from build123d import *

# Parameters (mm, degrees)
F0_W      = 120
F0_H      = 15
F1_DEPTH  = 781
F3_W      = 8
F3_H      = 8
F5_W      = 55
F5_H      = 12
F6_DEPTH  = 25
F7_W      = 20
F7_H      = 32
F9_DEPTH  = 25
F8_W      = 20
F8_H      = 32
F10_DEPTH = 25
F11_R     = 5


with BuildPart() as f1:
    # F0 (on Right) → F1 (new body)
    with BuildSketch(Plane.YZ):
        Rectangle(F0_W, F0_H)
    extrude(amount=F1_DEPTH)

    # F4: sweep along a path in F2
    with BuildLine(Plane.XY.offset(7.5)) as f4_path:
        Line((153, 60), (153, 10))
        ThreePointArc((153, 10), (155.928932, 2.928932), (163, 0))
        Line((163, 0), (553, 0))
        ThreePointArc((553, 0), (560.071068, 2.928932), (563, 10))
        Line((563, 10), (563, 60))
    # F3 (on face) → F4 (sweep, cut)
    with BuildSketch(Plane(origin=(0, 60, 0), x_dir=(-1, 0, 0), z_dir=(0, 1, 0))):
        with Locations((-152.987316, 11.5)):
            Rectangle(F3_W, F3_H)
        with Locations((-152.987316, 3.5)):
            Rectangle(F3_W, F3_H)
    sweep(path=f4_path.line, mode=Mode.SUBTRACT)

    # F5 (on face) → F6 (cut)
    with BuildSketch(Plane.XY.offset(7.5)):
        with Locations((152.987316, 60)):
            Rectangle(F5_W, F5_H)
        with Locations((563.012684, 60)):
            Rectangle(F5_W, F5_H)
    extrude(amount=-F6_DEPTH, mode=Mode.SUBTRACT)

    # F7 (on face) → F9 (cut)
    with BuildSketch(Plane.XY.offset(7.5)):
        with Locations((152.987316, 54)):
            Rectangle(F7_W, F7_H)
    extrude(amount=-F9_DEPTH, mode=Mode.SUBTRACT)

    # F8 (on face) → F10 (cut)
    with BuildSketch(Plane.XY.offset(7.5)):
        with Locations((563.012684, 54)):
            Rectangle(F8_W, F8_H)
    extrude(amount=-F10_DEPTH, mode=Mode.SUBTRACT)

    # F11
    f11_edges = [f1.edges().sort_by_distance(p)[0] for p in [
        (390.5, -60, -7.5),
        (390.5, -60, 7.5),
    ]]
    fillet(f11_edges, radius=F11_R)


solid = f1.part
The model under review builds one solid part; all positions refer to its coordinate system, in mm. A direction names the side the tool comes from. Round coordinates to 2 decimals unless told otherwise and drop trailing zeros. Write each loop counter-clockwise with the first axis right and the second up, starting at its lowest first coordinate (ties: lowest second). Pieces come first, ordered by that corner, then holes. Notation, with made-up numbers: (38, -27.75) - (70, -27.75) arc R32 cw to (70, 6.25) - close; hole circle Ø4 at (-28.5, -13.5). An arc over 180 degrees is marked (long way). One line per item, written item: value. Start each with the question number.
1. The part is to be moulded in two halves that separate along Y. For faces 1 (the face through (390, 1, -0.5)), 2 (the face through (153, 38, -2)), 3 (the face through (781, -1, 0)), say which applies: released by +Y, released by -Y, zero draft, split by the parting line, or undercut.
2. Consider section A-A on x = 543.5. Write out the cut boundary in (y, z), and give its area (3 significant figures).
3. Machinability: for faces 4 (the face through (562.799, -0.017, 3.556)), 5 (the face through (356, 60, 0)), 6 (the face through (563, 38, -2)), which of the approach directions +Z, -Z, +X, -X, +Y, -Y give a long, thin tool a straight path to every point of the face, cutting with its end or side? Answer none if there is none.
4. Consider section B-B on z = -5. Write out the cut boundary in (x, y), and give its area (3 significant figures).
5. Clearance check with a flat-ended pin moving along its axis: P1, Ø7.5, axis at x = 582.5, z = 1.5, coming from the +Y side. State where the tip first meets the part, or that it passes through.
6. To check wall thickness, follow L1, parallel to X at y = 41.5, z = -4.25; L2, parallel to X at y = 28, z = 2.5; L3, parallel to Y at x = 539, z = 5.75. State the ranges of each line that lie inside material, in increasing order. Write a range as from..to.
Checks:
1. face 1: undercut
1. face 2: released by +Y
1. face 3: zero draft
2. outline: (-60, -2.5) arc R5 ccw to (-55, -7.5) - (54, -7.5) - (54, 7.5) - (3.99, 7.5) - (3.99, -0.5) - (-4.01, -0.5) - (-4.01, 7.5) - (-55, 7.5) arc R5 ccw to (-60, 2.5) - close
2. area: 1,640 mm^2
3. face 4: +Z
3. face 5: +Z, -Z, +X, -X, +Y
3. face 6: +Z, -Z, +Y
4. outline: (0, -59.33) - (781, -59.33) - (781, 60) - (590.51, 60) - (590.51, 54) - (573.01, 54) - (573.01, 38) - (553.01, 38) - (553.01, 54) - (535.51, 54) - (535.51, 60) - (180.49, 60) - (180.49, 54) - (162.99, 54) - (162.99, 38) - (142.99, 38) - (142.99, 54) - (125.49, 54) - (125.49, 60) - (0, 60) - close
4. area: 91,900 mm^2
5. P1: stops at y = 54
6. L1: x = 0..142.99, 162.99..553.01, 573.01..781
6. L2: x = 0..148.99, 156.99..559.01, 567.01..781
6. L3: y = -58.8..-4.01, 3.99..54
